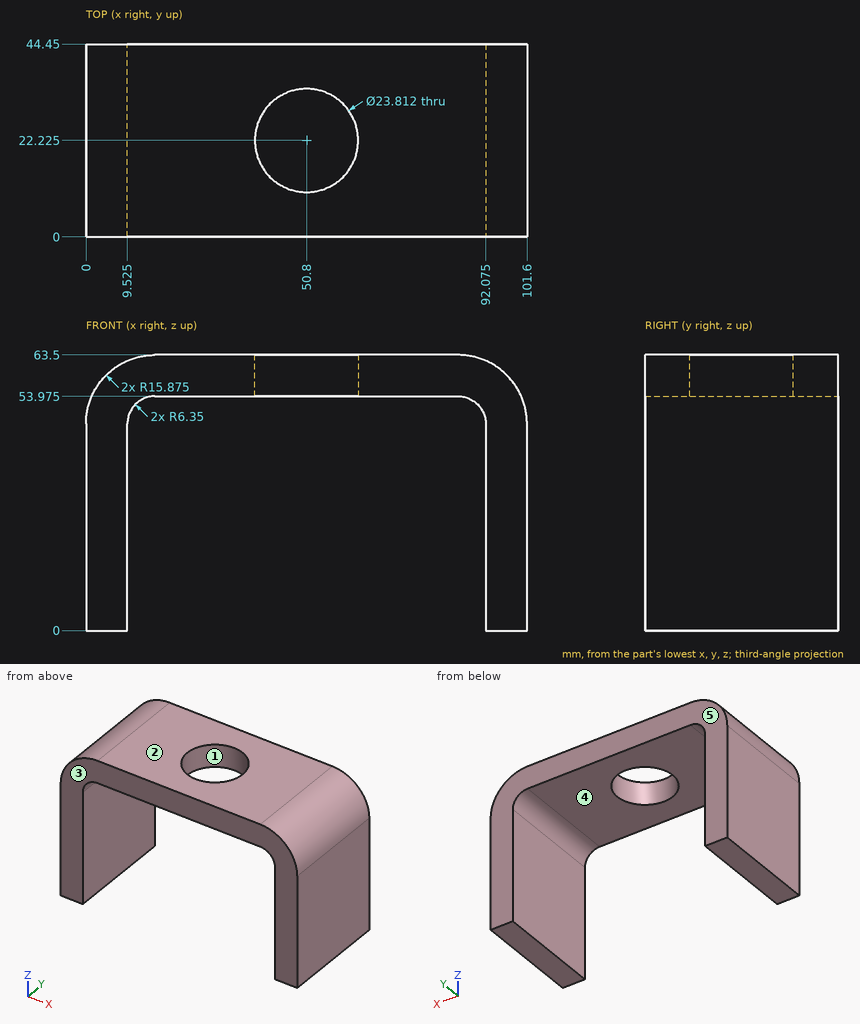
Geometry: see drawing. Coordinates: mm, zero at the bounding-box minimum. A direction names the side the tool comes from. Give positions to 0.01 mm unless a question says otherwise; leave off trailing zeros.
Q1. Draft query along Y for the marked faces 1, 2 and 3. Return one class per face: +Y half, -Y half, draft (parallel to the pull), parting line (faces both ways), or undercut.
Checked values:
face 1: undercut
face 2: draft
face 3: -Y half
Q2. Contact query for a flat-ended pin moving along its axis: pin 1 Ø13.5 at (x, y) = (38, 31.5) entering from -Z (1 decimal). Output: stop coordinate, or through.
Checked values:
pin 1: stops at z = 54
Q3. Ray query, probe 1 along X at (y, z) = (28, 31) (1 decimal); probe 2 along Y at (x, z) = (50.8, 59.25); probe 3 along X at (y, z) = (30.5, 60). Return the intervals inside material, ascending.
Checked values:
probe 1: x = 0 to 9.5, 92.1 to 101.6
probe 2: y = 0 to 10.32, 34.13 to 44.45
probe 3: x = 5.93 to 42.24, 59.36 to 95.67
Q4. Set-up query: the marked faces 4 and 5. Return all of +Z, -Z, +X, -X, +Y, -Y with unobstructed straight access to the full face (end or side cutting, diameter ignored); none if empty.
Checked values:
face 4: -Z, +Y, -Y
face 5: +Z, -Z, +X, -X, +Y
